The listing builds one solid part. Answer for the finished solid, in the listing's coordinates (mm). A direction names the side the tool comes from. Round coordinates to 2 decimals unless told otherwise and drop trailing zeros. Order: outer loops, then holes, each group sorted by start corner. A loop starts at its lowest first (then second) coordinate and runs counter-clockwise, first axis right, second up. Notation, with made-up numbers: M 9.25,-3 L 57.25,-3 A21 ccw 57.25,33 Z; hole C -7.75,7.5 d2. An arc over 180 degrees is marked long. Put each result on its own line as item: value. Start each with the question number.
1. The part is cut by section A-A (z = 22.25). Give the vertices of the cut face in (x, y), then the cut area to 3 significant figures.
2. Each of these flat-tipped pins is pushed along its axis until it touches: pin 1 Ø4 at (y, z) = (6, 25.5) entering from -X; pin 2 Ø1.6 at (y, z) = (16, 21.5) entering from +X; pin 3 Ø4 at (x, z) = (2, 5) entering from +Y; pin 4 Ø7.5 at (x, z) = (22, 16.5) entering from -Y. Where does it stop, or does it pass through?
3. The part is cut by section C-C (x = 15.5). Give the vertices of the cut face in (y, z).
4. The part is cut by section B-B (y = 5). Give the vertices of the cut face in (x, z).
5. Which of the six approach directions +Z, -Z, +X, -X, +Y, -Y give full straight-line access (tool end or side, diameter ignored) to faces 4 (the face through (1.69, 22.75, 8.1)), 5 (the face through (1.6, 18.6, 0.57)), 6 (the face through (1, 19.2, 24)), 7 (the face through (19.372, 8, 12)), 8 (the face through (12.372, 15, 15))?
6. The mould has two halves that part along X. Classify faces 1 (the face through (18.8, -2.4, 15.2)), 2 (the face through (14.372, 8, 11)), 3 (the face through (16.907, 6.64, 16.905)): +X half, -X half, draft (parallel to the pull), parting line (faces both ways), or undercut.
7. The part is cut by section D-D (z = 10.5). Give the vertices of the cut face in (x, y).
8. Consider line 1 (X direction, y = 5.75, z = 18.5); line 2 (Z direction, x = 16.3, y = 8.1); line 3 (X direction, y = 15, z = 11.75). Determine where each line is inside the solid, lowest interval first.
Autodesk Inventor part; units mm, degrees
ref_plane "YZ Plane" through (0, 0, 0) normal (1, 0, 0) x (0, 1, 0)
ref_plane "XZ Plane" through (0, 0, 0) normal (0, 1, 0) x (-1, 0, 0)
ref_plane "XY Plane" through (0, 0, 0) normal (0, 0, 1) x (1, 0, 0)
sketch "Skizze1" plane through (0, 0, 0) normal (0, 0, 1) x (1, 0, 0)
  line L0 (-14.1284, 0) -> (-14.1284, 16.2)
  line L1 (-14.1284, 16.2) -> (-12.1284, 16.2)
  line L2 (-12.1284, 16.2) -> (-12.1284, 1.6)
  line L3 (-12.1284, 1.6) -> (12.3716, 1.6)
  line L4 (12.3716, 1.6) -> (12.3716, 16.2)
  line L5 (12.3716, 16.2) -> (14.3716, 16.2)
  line L6 (14.3716, 16.2) -> (14.3716, 0)
  line L7 (14.3716, 0) -> (-14.1284, 0)
  line L8 (-16.6284, 19.2) -> (19.3716, 19.2)
  line L9 (19.3716, 19.2) -> (19.3716, -3)
  line L10 (19.3716, -3) -> (-16.6284, -3)
  line L11 (-16.6284, -3) -> (-16.6284, 19.2)
  line L12 (-12.1284, 14.7) -> (12.3716, 14.7)
  point P0 (0, 0)
  dimension "d1" = 2
  dimension "d3" = 2
  dimension "d4" = 1.6
  dimension "d5" = 3
  dimension "d7" = 2.5
  dimension "d8" = 5
  dimension "d9" = 1.5
  dimension "d26" = 3
  dimension "d27" = 28.5
  dimension "d28" = 16.2
extrude "Extrusion1" add sketch "Skizze1" along normal blind 30
fillet "Rundung1" radius 2 12 edges at (19.3716, 19.2, 15) (19.3716, -3, 15) (-16.6284, -3, 15) (-16.6284, 19.2, 15) (1.3716, 19.2, 30) (-16.6284, 8.1, 30) (1.3716, -3, 30) (19.3716, 8.1, 30) (19.3716, 8.1, 0) (1.3716, -3, 0) (1.3716, 19.2, 0) (-16.6284, 8.1, 0)
sketch "Skizze2" plane through (19.3716, -1, 28) normal (1, 0, 0) x (0, 0, -1)
  line L0 (0, 20.2) -> (26, 20.2)
  line L1 (8, 20.2) -> (4.25, 27.2)
  line L2 (4.25, 27.2) -> (21.75, 27.2)
  line L3 (21.75, 27.2) -> (18, 20.2)
  line L4 (28, 0) -> (28, 18.2)
  point P0 (28, 1)
  dimension "d13" = 10
  dimension "d15" = 7
  dimension "d16" = 3.75
  dimension "d17" = 3.75
  dimension "d18" = 17.5
  dimension "d19" = 10
extrude "Extrusion2" add sketch "Skizze2" against normal blind 41 and the other way blind 5
sketch "Skizze5" plane through (19.3716, -1, 28) normal (1, 0, 0) x (0, 0, -1)
  circle A0 centre (13, 9.1) radius 2.4
  line L0 (13, 9.1) -> (-2, 9.1)
  line L1 (-2, 18.2) -> (-2, 0)
  line L2 (13, 9.1) -> (13, 20.2)
  line L3 (8, 20.2) -> (18, 20.2)
  line L4 (13, 9.1) -> (28, 9.1)
  point P0 (28, 1)
  dimension "d31" = 4.8
  dimension "d32" = 90
  dimension "d35" = 15
extrude "Extrusion5" cut sketch "Skizze5" against normal blind 10
properties part number "7.2 Schienenläufer"
Resolved:
1. outline: M -21.63,23.4 L 24.37,23.4 L 24.37,26.2 L -21.63,26.2 Z; M -16.63,-1 A2 ccw -14.63,-3 L 17.37,-3 A2 ccw 19.37,-1 L 19.37,17.2 A2 ccw 17.37,19.2 L -14.63,19.2 A2 ccw -16.63,17.2 Z; hole M -14.13,0 L 14.37,0 L 14.37,16.2 L 12.37,16.2 L 12.37,14.7 L -12.13,14.7 L -12.13,16.2 L -14.13,16.2 Z
1. area: 500 mm2
2. pin 1: x = -16.63
2. pin 2: x = 19.37
2. pin 3: y = 26.2
2. pin 4: y = -2.8
3. outline: M -3,2 A2 ccw -1,0 L 17.2,0 A2 ccw 19.2,2 L 19.2,10 L 26.2,6.25 L 26.2,23.75 L 19.2,20 L 19.2,28 A2 ccw 17.2,30 L -1,30 A2 ccw -3,28 Z; hole C 8.1,15 d4.8
4. outline: M -16.63,2 A2 ccw -14.63,0 L -14.13,0 L -14.13,30 L -14.63,30 A2 ccw -16.63,28 Z; M 14.37,0 L 17.37,0 A2 ccw 19.37,2 L 19.37,28 A2 ccw 17.37,30 L 14.37,30 Z
5. face 4: -Z, +X, -X
5. face 5: -Z, +X, -X, +Y
5. face 6: +Z, +X, -X
5. face 7: +Z, -Z, +X, -Y
5. face 8: +Z, -Z
6. face 1: +X half
6. face 2: undercut
6. face 3: draft
7. outline: M -21.63,19.2 L -14.63,19.2 A2 ccw -16.63,17.2 L -16.63,-1 A2 ccw -14.63,-3 L 17.37,-3 A2 ccw 19.37,-1 L 19.37,17.2 A2 ccw 17.37,19.2 L 24.37,19.2 L 24.37,26.2 L -21.63,26.2 Z; hole M -14.13,0 L 14.37,0 L 14.37,16.2 L 12.37,16.2 L 12.37,14.7 L -12.13,14.7 L -12.13,16.2 L -14.13,16.2 Z
8. line 1: -16.63 to -14.13, 14.37 to 19.37
8. line 2: 0 to 12.6, 17.4 to 30
8. line 3: -16.63 to -14.13, -12.13 to 12.37, 14.37 to 19.37
